For this review, take the finished solid that the model builds, in its own axes (mm). A direction names the side the tool comes from. Round coordinates to 2 decimals unless told otherwise and drop trailing zeros. Order: outer loops, then holes, each group sorted by start corner. A loop starts at its lowest first (then second) coordinate and runs counter-clockwise, first axis right, second up. Notation, with made-up numbers: (84.5, 31.5) - (93.5, 31.5) arc R25 ccw to (93.5, 51.5) - close; hole circle Ø10 at (42.5, 88.5). An arc over 180 degrees is marked (long way). Write each question's results on one line, items separated by ' | '. Start each with the question number.
(1) Take a section at D-D, the plane x = 4.5. Give the boundary of the cut face in (y, z) (3 decimals).
(2) Draft analysis for pull direction X (two halves, no side actions). For faces 1 (the flat face through (-9.75, -1, 0)), 2 (the flat face through (0, 70.8, 0)), 3 (the flat face through (0, 73.6, -2.1)), state which applies: pulls with the +X half, pulls with the -X half, needs draft (parallel to the pull), parting line crosses it, or undercut.
(3) Take a section at C-C, the plane y = 25. Give the boundary of the cut face in (x, z) (3 decimals), plus the area to 3 significant figures.
(4) Take a section at A-A, the plane z = 0. Give the boundary of the cut face in (x, y) (3 decimals), plus the area to 3 significant figures.
(5) Insertion check: pin 1 Ø4 at (x, y) = (-5.5, 17.5) entering from -Z; pin 2 Ø1.5 at (y, z) = (60, -0.5) entering from -X (3 decimals); pin 3 Ø6 at (x, y) = (3.5, 25) entering from +Z; pin 4 Ø1.5 at (x, y) = (3.5, 15) entering from +Z. Each pin has a flat end and moves straight along its axis. Give the tip position at first contact, or say it passes through.
(6) For faces 4 (the cylindrical face through (0.426, 36.285, -3.247)), 5 (the flat face through (0, 74.6, 0)), 6 (the cylindrical face through (-1.9, 35.03, -0.08)), list the 3-axis set-ups (+Z, -Z, +X, -X, +Y, -Y) from which the entire face can be reached by the end or side of a thin tool; tool diameter is ignored.
(7) For L1, parallel to Z at x = 0, y = 55 (3 decimals); L2, parallel to Y at x = -3, z = -1; L3, parallel to Y at x = -5, z = 3, list the stretches that pass through material, from the lowest coordinate up. Write a range as from..to.
(8) Take a section at B-B, the plane x = 0. Give the boundary of the cut face in (y, z) (3 decimals), plus the area to 3 significant figures.
Autodesk Inventor part; units mm, degrees
ref_plane "YZ Plane" through (0, 0, 0) normal (1, 0, 0) x (0, 1, 0)
ref_plane "XZ Plane" through (0, 0, 0) normal (0, 1, 0) x (-1, 0, 0)
ref_plane "XY Plane" through (0, 0, 0) normal (0, 0, 1) x (1, 0, 0)
sketch "Sketch1" plane through (0, 0, 0) normal (0, 1, 0) x (-1, 0, 0)
  circle A0 centre (0, 0) radius 3.275
  dimension "d0" = 6.55
extrude "Extrusion1" add sketch "Sketch1" along normal blind 73.6
sketch "Sketch2" plane through (0, 0, 0) normal (0, -1, 0) x (1, 0, 0)
  circle A0 centre (0, 0) radius 1.9
  dimension "d3" = 3.8
extrude "Extrusion2" cut sketch "Sketch2" against normal blind 70.8
sketch "Sketch3" plane through (0, 73.6, 0) normal (0, 1, 0) x (1, 0, 0)
  circle A0 centre (0, 0) radius 1.9
extrude "Extrusion3" add sketch "Sketch3" along normal blind 1
sketch "Sketch4" plane through (0, 0, 0) normal (0, -1, 0) x (1, 0, 0)
  line L0 (0, 0) -> (0, 4.725)
  line L1 (0, 4.725) -> (0, -4.725)
  line L2 (0, 4.725) -> (9.75, 4.725)
  line L3 (9.75, 4.725) -> (-9.75, 4.725)
  line L4 (-9.75, 4.725) -> (-9.75, -4.725)
  line L5 (-9.75, -4.725) -> (9.75, -4.725)
  line L6 (9.75, -4.725) -> (9.75, 4.725)
  circle A0 centre (0, 0) radius 1.9
  dimension "d8" = 4.725
  dimension "d9" = 9.45
  dimension "d10" = 9.75
  dimension "d11" = 19.5
extrude "Extrusion4" add sketch "Sketch4" along normal blind 1.75 contours A0 L1 L5 L4 L3 L0 | L0 L2 L6 L5 L1 A0
properties part number "SyringeBody"
Results below:
1) outline: (-1.75, -4.725) - (0, -4.725) - (0, 4.725) - (-1.75, 4.725) - close
2) face 1: pulls with the -X half | face 2: undercut | face 3: needs draft
3) outline: circle Ø6.55 at (0, 0); hole circle Ø3.8 at (0, 0) | area: 22.4 mm^2
4) outline: (-9.75, -1.75) - (-1.9, -1.75) - (-1.9, 70.8) - (1.9, 70.8) - (1.9, -1.75) - (9.75, -1.75) - (9.75, 0) - (3.275, 0) - (3.275, 73.6) - (1.9, 73.6) - (1.9, 74.6) - (-1.9, 74.6) - (-1.9, 73.6) - (-3.275, 73.6) - (-3.275, 0) - (-9.75, 0) - close | area: 244 mm^2
5) pin 1: passes through | pin 2: stops at x = -3.275 | pin 3: stops at z = 3.24 | pin 4: stops at z = 1.78
6) face 4: +Y | face 5: +Z, -Z, +X, -X, +Y | face 6: -Y
7) L1: z = -3.275..-1.9, 1.9..3.275 | L2: y = -1.75..73.6 | L3: y = -1.75..0
8) outline: (-1.75, -4.725) - (0, -4.725) - (0, -3.275) - (73.6, -3.275) - (73.6, -1.9) - (74.6, -1.9) - (74.6, 1.9) - (73.6, 1.9) - (73.6, 3.275) - (0, 3.275) - (0, 4.725) - (-1.75, 4.725) - (-1.75, 1.9) - (70.8, 1.9) - (70.8, -1.9) - (-1.75, -1.9) - close | area: 227 mm^2
